Verification items for the finished model (mm, model axes). Face numbers are marked on the shaded views. A direction names the side the tool comes from. Coordinates: 2 decimals unless noted, no trailing zeros. Loops run counter-clockwise (first coordinate to the right, second up) from the corner with the lowest first, then second, coordinate; pieces in that order, holes last. Notation, with made-up numbers: M -39,-7 L -10,-7 A32 cw -10,21 Z; hole C -13.5,69.5 d10. An arc over 180 degrees is marked long. Write item = value, one per line. Start each with the question number.
```python
from build123d import *

# Parameters (mm, degrees)
SKETCH_1_R      = 1.45
EXTRUDE_1_DEPTH = 3
FILLET_1_R      = 4


with BuildPart() as part:
    # 草图1 → 凸台-拉伸1 (new body)
    with BuildSketch(Plane.XY):
        Polygon((-6, 6), (-25, 6), (-25, -6), (25, -6), (25, 6), (6, 6), (6, 41), (-6, 41), align=None)
        with Locations((0, 35)):
            Circle(SKETCH_1_R, mode=Mode.SUBTRACT)
        Circle(SKETCH_1_R, mode=Mode.SUBTRACT)
        with Locations((-20, 0)):
            Circle(SKETCH_1_R, mode=Mode.SUBTRACT)
        with Locations((20, 0)):
            Circle(SKETCH_1_R, mode=Mode.SUBTRACT)
        with Locations((0, 15)):
            Circle(SKETCH_1_R, mode=Mode.SUBTRACT)
    extrude(amount=EXTRUDE_1_DEPTH)

    # 圆角1
    fillet_1_edges = [part.edges().sort_by_distance(p)[0] for p in [
        (-6, 41, 1.5),
        (6, 41, 1.5),
        (6, 6, 1.5),
        (25, 6, 1.5),
        (25, -6, 1.5),
        (-25, -6, 1.5),
        (-25, 6, 1.5),
        (-6, 6, 1.5),
    ]]
    fillet(fillet_1_edges, radius=FILLET_1_R)


solid = part.part
```
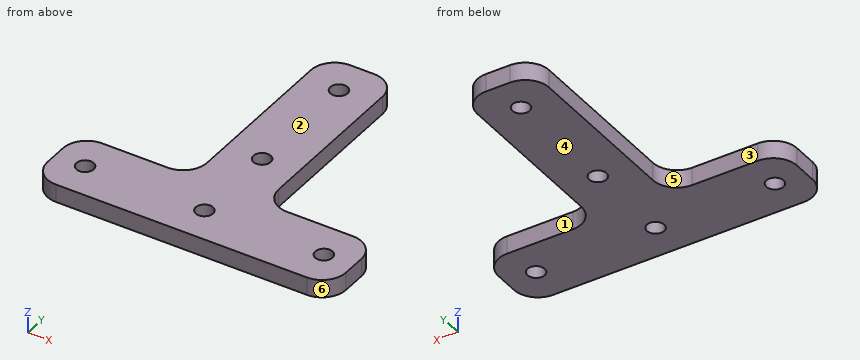
Q1. Set-up check for the marked faces 1, 2 and 3: record each of +Z, -Z, +X, -X, +Y, -Y from which the full face is reachable in a straight line by a thin tool's end or side.
Q2. Scan lines: L1, parallel to Y at x = 0, z = 0.95; L2, parallel to X at y = -0.5, z = 2; L3, parallel to Y at x = 20, z = 0.7. Record each from-to range of solid material in increasing order. Write a range as [from, to].
Q3. Gauge pin test, flat ends, axial feed: pin 1 (1.7 mm diameter, centred on x = 0, y = 15, fed in from -Z); pin 2 (1.5 mm diameter, centred on x = -14.5, z = 1.5, fed in from +Y). Record the tip position at first contact, or that the pin passes through.
Q4. Mould release check, pull along X, two halves, no side actions. Record for the marked faces 4, 5 and 6: +X half, -X half, draft (parallel to the pull), parting line (faces both ways), or undercut.
Q5. Sectioned sample at B-B on y = 0. Record the cut outline in (x, z), plus the area to 3 significant figures.
Q6. Sectioned sample at C-C on z = 1. Record the cut outline in (x, y), plus the area to 3 significant figures.
Q7. Sectioned sample at A-A on y = 35. Record the cut outline in (x, z).
Solutions:
q1.face_1 = +Z, -Z, +X, +Y
q1.face_2 = +Z, +X, -X, +Y, -Y
q1.face_3 = +Z, -Z, -X, +Y
q2.L1 = [-6, -1.45], [1.45, 13.55], [16.45, 33.55], [36.45, 41]
q2.L2 = [-25, -21.36], [-18.64, -1.36], [1.36, 18.64], [21.36, 25]
q2.L3 = [-6, -1.45], [1.45, 6]
q3.pin_1 = through
q3.pin_2 = 6
q4.face_4 = draft
q4.face_5 = -X half
q4.face_6 = +X half
q5.outline = M -25,0 L -21.45,0 L -21.45,3 L -25,3 Z; M -18.55,0 L -1.45,0 L -1.45,3 L -18.55,3 Z; M 1.45,0 L 18.55,0 L 18.55,3 L 1.45,3 Z; M 21.45,0 L 25,0 L 25,3 L 21.45,3 Z
q5.area = 124 mm²
q6.outline = M -25,-2 A4 ccw -21,-6 L 21,-6 A4 ccw 25,-2 L 25,2 A4 ccw 21,6 L 10,6 A4 cw 6,10 L 6,37 A4 ccw 2,41 L -2,41 A4 ccw -6,37 L -6,10 A4 cw -10,6 L -21,6 A4 ccw -25,2 Z; hole C -20,0 d2.9; hole C 0,0 d2.9; hole C 0,15 d2.9; hole C 0,35 d2.9; hole C 20,0 d2.9
q6.area = 973 mm²
q7.outline = M -6,0 L -1.45,0 L -1.45,3 L -6,3 Z; M 1.45,0 L 6,0 L 6,3 L 1.45,3 Z
